Read the model definition and answer for the solid it produces. Units are mm, in the model's axes. Face numbers are marked on the shaded views. A direction names the side the tool comes from. Give positions to 0.01 mm unless a question says otherwise; leave off trailing zeros. Order: outer loops, then holes, each group sorted by start corner. A loop starts at its lowest first (then second) coordinate and runs counter-clockwise, first axis right, second up. Notation, with made-up numbers: (12.5, -2.5) - (60.5, -2.5) arc R31 cw to (60.5, 24.5) - close; hole circle Ø1 at (42.5, 11.5). An arc over 180 degrees is marked (long way). One line per item, written item: value. Start each with the question number.
```python
from build123d import *

# Parameters (mm, degrees)
SKETCH2_W           = 186.37
SKETCH2_H           = 200
BOSS_EXTRUDE2_DEPTH = 900
SKETCH3_W           = 70
SKETCH3_H           = 200
BOSS_EXTRUDE3_DEPTH = 60
SKETCH4_W           = 1400
SKETCH4_H           = 550
BOSS_EXTRUDE4_DEPTH = 50
CUT_EXTRUDE1_DEPTH  = 900
SKETCH7_W           = 900
SKETCH7_H           = 15
BOSS_EXTRUDE5_DEPTH = 30
SKETCH8_W           = 760
SKETCH8_H           = 15
BOSS_EXTRUDE6_DEPTH = 30


with BuildPart() as part:
    # Sketch2 → Boss-Extrude2 (new body)
    with BuildSketch(Plane(origin=(0, 0, 0), x_dir=(0, 0, -1), z_dir=(1, 0, 0))):
        Rectangle(SKETCH2_W, SKETCH2_H)
    extrude(amount=-BOSS_EXTRUDE2_DEPTH)

    # Sketch3 → Boss-Extrude3 (add)
    with BuildSketch(Plane.XY.offset(93.185)):
        with Locations((-35, 0)):
            Rectangle(SKETCH3_W, SKETCH3_H)
        with Locations((-865, 0)):
            Rectangle(SKETCH3_W, SKETCH3_H)
    extrude(amount=BOSS_EXTRUDE3_DEPTH)

    # Sketch4 → Boss-Extrude4 (add)
    with BuildSketch(Plane.XZ.offset(100)):
        with Locations((-580, 61.815)):
            Rectangle(SKETCH4_W, SKETCH4_H)
    extrude(amount=BOSS_EXTRUDE4_DEPTH)

    # Sketch6 → Cut-Extrude1 (cut)
    with BuildSketch(Plane(origin=(0, 0, 0), x_dir=(0, 0, -1), z_dir=(1, 0, 0))):
        with BuildLine():
            Line((-44.815, 100), (-44.815, 81.242091756))
            add(Edge.make_bspline(
                [(-44.815, 81.242091756), (15.185, 17.399871026), (75.185, 81.242091756)],
                knots=[0, 0, 0, 1, 1, 1], degree=2))
            Line((75.185, 81.242091756), (75.185, 100))
            Line((75.185, 100), (-44.815, 100))
        make_face()
    extrude(amount=-CUT_EXTRUDE1_DEPTH, mode=Mode.SUBTRACT)

    # Sketch7 → Boss-Extrude5 (add)
    with BuildSketch(Plane(origin=(0, 0, -93.185), x_dir=(-1, 0, 0), z_dir=(0, 0, -1))):
        with Locations((450, 92.5)):
            Rectangle(SKETCH7_W, SKETCH7_H)
    extrude(amount=BOSS_EXTRUDE5_DEPTH)

    # Sketch8 → Boss-Extrude6 (add)
    with BuildSketch(Plane.XY.offset(93.185)):
        with Locations((-450, 92.5)):
            Rectangle(SKETCH8_W, SKETCH8_H)
    extrude(amount=BOSS_EXTRUDE6_DEPTH)


solid = part.part
```
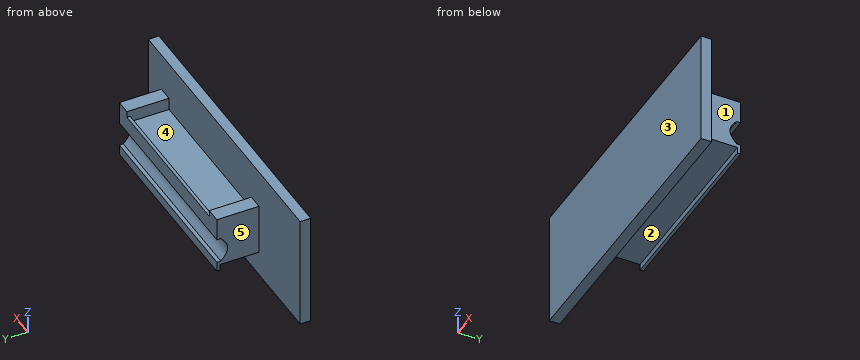
1) Find the intervals of material crossed by probe 1 along X at (y, z) = (-75.5, 136.5); probe 2 along Y at (x, z) = (-320.5, -107); probe 3 along Y at (x, z) = (-890, -175.5), in increasing order. Write a range as from..to.
2) The mould has two halves that part along Y. Classify the marked faces 3, 4 and 5: +Y half, -Y half, draft (parallel to the pull), parting line (faces both ways), or undercut.
3) Section D-D on z = -160.5 is taken. Write down the section's boundary in (x, y).
4) For the marked faces 1 and 2, determine the directions among +Z, -Z, +X, -X, +Y, -Y from which every point of the face is accessible in a straight line to the end or side of a thin tool.
5) Section C-C on x = -1092 is taken. Write down the section's boundary in (y, z) (3 decimals), plus the area to 3 significant figures.
6) Section B-B on y = -41 is taken. Write down the section's boundary in (x, z) (3 decimals).
7) Section A-A on z = 68.5 is taken. Write down the section's boundary in (x, y).
8) Each of these flat-tipped pins is pushed along its axis until it touches: pin 1 (2 mm diameter, centred on x = -726, y = 19.5, fed in from +Z) (3 decimals); pin 2 (1.5 mm diameter, centred on x = -292.5, y = -6, fed in from -Z) (3 decimals); pin 3 (3 mm diameter, centred on y = -59, z = 126.5, fed in from -X). Where does it stop, or does it pass through?
Solved:
1. probe 1: x = -900..-830, -70..0
1. probe 2: y = -150..-100, 85..100
1. probe 3: y = -150..-100
2. face 3: -Y half
2. face 4: undercut
2. face 5: draft
3. outline: (-1280, -150) - (120, -150) - (120, -100) - (-1280, -100) - close
4. face 1: +Z, -Z, +X, +Y
4. face 2: -Z, +X, -X
5. outline: (-150, -213.185) - (-100, -213.185) - (-100, 336.815) - (-150, 336.815) - close
5. area: 27,500 mm2
6. outline: (-900, -93.185) - (0, -93.185) - (0, 153.185) - (-70, 153.185) - (-70, 93.185) - (-830, 93.185) - (-830, 153.185) - (-900, 153.185) - close
7. outline: (-1280, -150) - (120, -150) - (120, -100) - (0, -100) - (0, 100) - (-900, 100) - (-900, -100) - (-1280, -100) - close
8. pin 1: stops at z = 93.185
8. pin 2: stops at z = -93.185
8. pin 3: stops at x = -900
